Here's the drawing with two shaded views (mm, measured from the low corner). I have some questions. Give positions to 0.01 mm unless a question says otherwise; leave off trailing zeros. Loops run counter-clockwise (first coordinate to the right, second up) from the corner with the lowest first, then second, coordinate; pieces in that order, holes last.
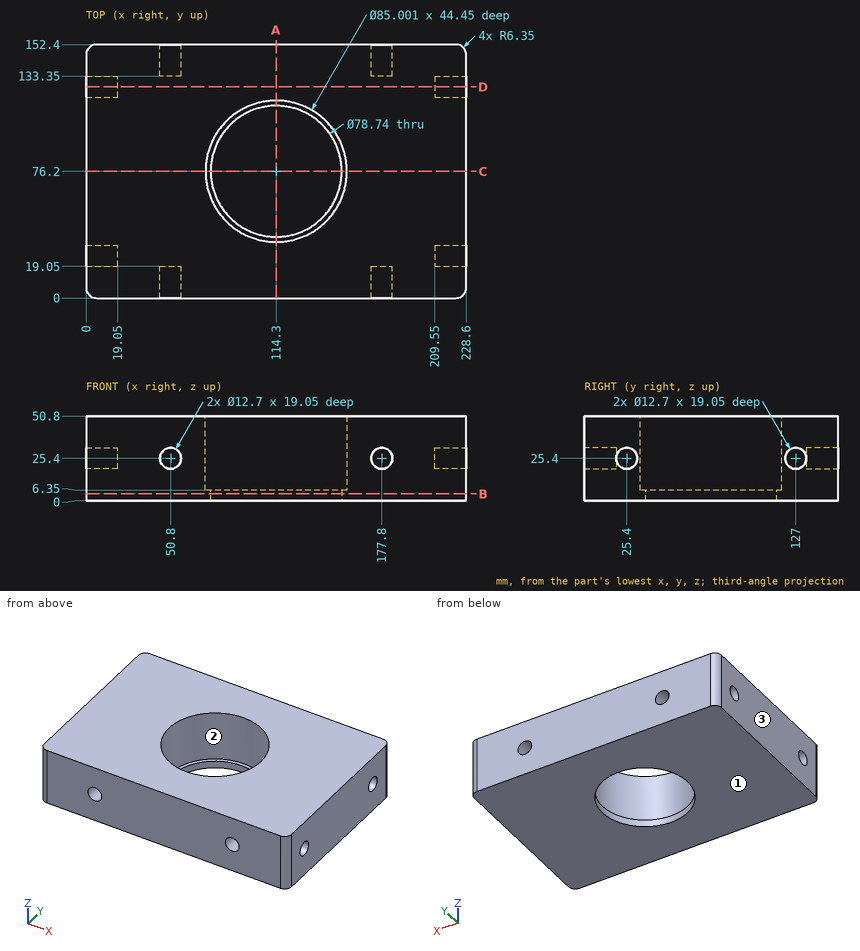
(1) Please list where these lines run through material, in increasing order: probe 1 along Y at (x, z) = (13, 25); probe 2 along Z at (x, y) = (177.8, 146); probe 3 along Y at (x, z) = (114.3, 2.25).
Returned:
probe 1: y = 0 to 19.06, 31.74 to 120.66, 133.34 to 152.4
probe 2: z = 0 to 19.05, 31.75 to 50.8
probe 3: y = 0 to 36.83, 115.57 to 152.4
(2) Will these pins go through, and if not, where does the flat tip stop? P1, Ø6.5, axis at y = 22.5, z = 25.5, coming from the -X side; P2, Ø11.5, axis at x = 50.8, z = 25.4, coming from the +Y side; P3, Ø6.5, axis at x = 52.5, z = 26, coming from the -Y side.
Returned:
P1: stops at x = 19.05
P2: stops at y = 133.35
P3: stops at y = 19.05
(3) Suppose I cut it at C-C on y = 76.2. List the corners of the cut face in (x, z) for me, plus the area to 3 significant figures.
Returned:
outline: (0, 0) - (74.93, 0) - (74.93, 6.35) - (71.8, 6.35) - (71.8, 50.8) - (0, 50.8) - close; (153.67, 0) - (228.6, 0) - (228.6, 50.8) - (156.8, 50.8) - (156.8, 6.35) - (153.67, 6.35) - close
area: 7,330 mm2
(4) Suppose I cut it at D-D on y = 127. List the corners of the cut face in (x, z) for me.
Returned:
outline: (0, 0) - (228.6, 0) - (228.6, 19.05) - (209.55, 19.05) - (209.55, 31.75) - (228.6, 31.75) - (228.6, 50.8) - (0, 50.8) - (0, 31.75) - (19.05, 31.75) - (19.05, 19.05) - (0, 19.05) - close
(5) Thinking about a two-plate mould opening in X: for the marked faces 1, 2 and 3, which applies, pulls with the +X half, pulls with the -X half, needs draft (parallel to the pull), parting line crosses it, or undercut?
Returned:
face 1: needs draft
face 2: undercut
face 3: pulls with the -X half
(6) Suppose I cut it at A-A on x = 114.3. List the corners of the cut face in (y, z) for me, plus the area to 3 significant figures.
Returned:
outline: (0, 0) - (36.83, 0) - (36.83, 6.35) - (33.7, 6.35) - (33.7, 50.8) - (0, 50.8) - close; (115.57, 0) - (152.4, 0) - (152.4, 50.8) - (118.7, 50.8) - (118.7, 6.35) - (115.57, 6.35) - close
area: 3,460 mm2
(7) Suppose I cut it at B-B on z = 4. List the corners of the cut face in (x, y) for me, plus the area to 3 significant figures.
Returned:
outline: (0, 6.35) arc R6.35 ccw to (6.35, 0) - (222.25, 0) arc R6.35 ccw to (228.6, 6.35) - (228.6, 146.05) arc R6.35 ccw to (222.25, 152.4) - (6.35, 152.4) arc R6.35 ccw to (0, 146.05) - close; hole circle Ø78.74 at (114.3, 76.2)
area: 29,900 mm2
